Model file for the job. Use its own axes, mm. A direction names the side the tool comes from. Coordinates: 2 decimals unless noted, no trailing zeros. Order: outer loops, then holes, each group sorted by start corner. A loop starts at its lowest first (then second) coordinate and runs counter-clockwise, first axis right, second up. Notation, with made-up numbers: M -26,60 L 32,60 A19 cw 32,93 Z; hole C -24,-34 d8. An arc over 180 degrees is marked long. Return JSON: item names as keys, results as strings.
```python
from build123d import *

# Parameters (mm, degrees)
F0_W     = 50.8
F0_H     = 12.7
F0_W_2   = 12.7
F0_H_2   = 50.8
F1_DEPTH = 25.4
F2_D     = 12.7


with BuildPart() as f1:
    # F0 (on Top) → F1 (new body)
    with BuildSketch(Plane.XY):
        with Locations((38.1, -6.35)):
            Rectangle(F0_W, F0_H)
        with Locations((6.35, -38.1)):
            Rectangle(F0_W_2, F0_H_2)
        with Locations((6.35, -6.35)):
            Rectangle(F0_W_2, F0_H)
        with Locations((38.1, 6.35)):
            Rectangle(F0_W, F0_H)
        with Locations((-6.35, -38.1)):
            Rectangle(F0_W_2, F0_H_2)
        with Locations((-6.35, -6.35)):
            Rectangle(F0_W_2, F0_H)
        with Locations((6.35, 6.35)):
            Rectangle(F0_W_2, F0_H)
        with Locations((-38.1, -6.35)):
            Rectangle(F0_W, F0_H)
        with Locations((-6.35, 6.35)):
            Rectangle(F0_W_2, F0_H)
        with Locations((6.35, 38.1)):
            Rectangle(F0_W_2, F0_H_2)
        with Locations((-38.1, 6.35)):
            Rectangle(F0_W, F0_H)
        with Locations((-6.35, 38.1)):
            Rectangle(F0_W_2, F0_H_2)
    extrude(amount=F1_DEPTH)

    # F2 (through all)
    with Locations(Plane(origin=(0, 0, 0), x_dir=(1, 0, 0), z_dir=(0, 0, -1))):
        with Locations((31.75, 0), (0, -31.75), (-31.75, 0), (0, 0), (0, 31.75)):
            Hole(F2_D / 2)


solid = f1.part
```
Item 1: Wall check: line 1 (Y direction, x = 0, z = 11.5); line 2 (X direction, y = -31.75, z = 14.5); line 3 (X direction, y = -2.5, z = 11). Give the ranges that are in metal, low to high.
Check result:
{"line 1": "y = -63.5 to -38.1, -25.4 to -6.35, 6.35 to 25.4, 38.1 to 63.5", "line 2": "x = -12.7 to -6.35, 6.35 to 12.7", "line 3": "x = -63.5 to -37.59, -25.91 to -5.84, 5.84 to 25.91, 37.59 to 63.5"}
Item 2: Saw through at C-C (z = 12.25). Write the cut outline in (x, y), and give its area (3 significant figures).
Check result:
{"outline": "M -63.5,-12.7 L -12.7,-12.7 L -12.7,-63.5 L 12.7,-63.5 L 12.7,-12.7 L 63.5,-12.7 L 63.5,12.7 L 12.7,12.7 L 12.7,63.5 L -12.7,63.5 L -12.7,12.7 L -63.5,12.7 Z; hole C -31.75,0 d12.7; hole C 0,-31.75 d12.7; hole C 0,0 d12.7; hole C 0,31.75 d12.7; hole C 31.75,0 d12.7", "area": "5,170 mm2"}
Item 3: Saw through at A-A (x = 0). Write the cut outline in (y, z).
Check result:
{"outline": "M -63.5,0 L -38.1,0 L -38.1,25.4 L -63.5,25.4 Z; M -25.4,0 L -6.35,0 L -6.35,25.4 L -25.4,25.4 Z; M 6.35,0 L 25.4,0 L 25.4,25.4 L 6.35,25.4 Z; M 38.1,0 L 63.5,0 L 63.5,25.4 L 38.1,25.4 Z"}
Item 4: 3-axis set-ups, long thin cutter, end or side, ignore diameter. For faces 1 (the flat face through (-12.7, 38, 13)), 2 (the flat face through (-12.7, -38, 13)), 3 (the flat face through (38, 12.7, 13)): which of +Z, -Z, +X, -X, +Y, -Y reach the whole face in a straight line?
Check result:
{"face 1": "+Z, -Z, -X, +Y", "face 2": "+Z, -Z, -X, -Y", "face 3": "+Z, -Z, +X, +Y"}
Item 5: Drop flat-ended pins along their axis: pin 1 Ø10 at (x, y) = (0, 31.75) entering from +Z; pin 2 Ø7.5 at (y, z) = (-45, 18) entering from -X; pin 3 Ø6 at (x, z) = (-29.5, 11) entering from -Y; pin 4 Ø7.5 at (y, z) = (-47, 19) entering from +X. Give the stop position or say it passes through.
Check result:
{"pin 1": "passes through", "pin 2": "stops at x = -12.7", "pin 3": "stops at y = -12.7", "pin 4": "stops at x = 12.7"}
Item 6: Pull direction Y, two halves, no side cores. Call faces 4 (the flat face through (12.7, -38, 13)), 5 (the cylindrical face through (1.38, 6.2, 12.88)), 6 (the flat face through (38, -12.7, 13)): +Y half, -Y half, draft (parallel to the pull), parting line (faces both ways), or undercut.
Check result:
{"face 4": "draft", "face 5": "undercut", "face 6": "-Y half"}
Item 7: Saw through at B-B (y = -31.75). Write the cut outline in (x, z), and give its area (3 significant figures).
Check result:
{"outline": "M -12.7,0 L -6.35,0 L -6.35,25.4 L -12.7,25.4 Z; M 6.35,0 L 12.7,0 L 12.7,25.4 L 6.35,25.4 Z", "area": "323 mm2"}
